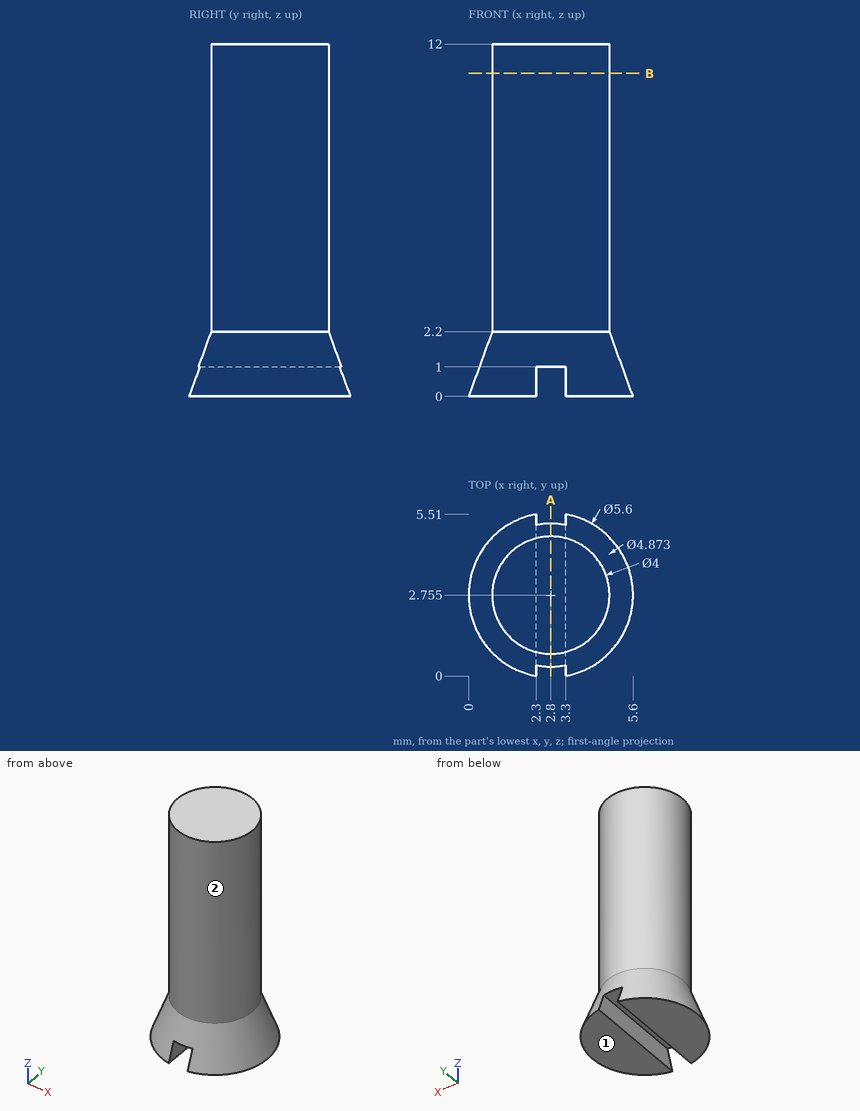
Here's the drawing with two shaded views (mm, measured from the low corner). I have some questions. A direction names the side the tool comes from. Coordinates: 2 decimals unless noted, no trailing zeros. Order: outer loops, then holes, each group sorted by start corner. A loop starts at its lowest first (then second) coordinate and runs counter-clockwise, first axis right, second up. Notation, with made-up numbers: (-39, 32.5) - (-1, 32.5) arc R9 cw to (-1, 38.5) - close; hole circle Ø8 at (47.5, 84.5). An arc over 180 degrees is marked (long way). Answer in a Markdown table with one row per item.
1. For pin 1 (3 mm diameter, centred on x = 4, z = 6, fed in from -Y) (3 decimals); pin 2 (2 mm diameter, centred on y = 2.5, z = 6, fed in from -X); pin 3 (1.1 mm diameter, centred on y = 3.5, z = 0.5, fed in from +X); pin 4 (0.8 mm diameter, centred on x = 2.5, y = 2, fed in from -Z), each with a flat end and sliding along its axis, tell me the tip position at first contact or that it passes through.
Reply:
| item | result |
|---|---|
| pin 1 | stops at y = 0.755 |
| pin 2 | stops at x = 0.8 |
| pin 3 | stops at x = 5.55 |
| pin 4 | stops at z = 0 |
2. Suppose I cut it at A-A (x = 2.8). Please give me the cut outline in (y, z) (1 decimal).
Reply:
| item | result |
|---|---|
| outline | (0.3, 1) - (5.2, 1) - (4.8, 2.2) - (4.8, 12) - (0.8, 12) - (0.8, 2.2) - close |
3. Suppose I cut it at B-B (z = 11). Please give me the cut outline in (x, y) (1 decimal).
Reply:
| item | result |
|---|---|
| outline | circle Ø4 at (2.8, 2.8) |
4. For the marked faces 1 and 2, which set-ups out of +Z, -Z, +X, -X, +Y, -Y let a thin tool reach every point of the face, with its end or its side?
Reply:
| item | result |
|---|---|
| face 1 | -Z, +X, -X, +Y, -Y |
| face 2 | +Z |
5. If I drill on line 1 along Z through (x, y) = (2.45, 2.3); line 2 along Y through (x, z) = (2.7, 5); line 3 along Y through (x, z) = (3.1, 5), over which ranges is the centre line in solid material (lowest first)?
Reply:
| item | result |
|---|---|
| line 1 | z = 1 to 12 |
| line 2 | y = 0.76 to 4.75 |
| line 3 | y = 0.78 to 4.73 |
